from build123d import *

# Parameters (mm, degrees)
EXTRUDE_1_DEPTH     = 12.2
SKETCH_3_W          = 3.6
SKETCH_3_H          = 1.2
CUT_EXTRUDE_1_DEPTH = 2
SKETCH_4_R          = 6.1
SKETCH_4_R_2        = 2.75
EXTRUDE_2_DEPTH     = 4.4
SKETCH_4_3_W        = 6.5
SKETCH_4_3_H        = 9.8
CUT_EXTRUDE_2_DEPTH = 0.2
SKETCH_5_R          = 2.4
SKETCH_5_R_2        = 0.9
EXTRUDE_3_DEPTH     = 3.4
CUT_EXTRUDE_3_REACH = 29.316


with BuildPart() as part:
    # Sketch 1 → Extrude 1 (new body)
    with BuildSketch(Plane.XY):
        Polygon((-11.25, 0), (11.25, 0), (11.25, 15.8), (16.2, 15.8), (16.2, 18.3), (11.25, 18.3), (11.25, 22.3), (-11.25, 22.3), (-11.25, 18.3), (-16.2, 18.3), (-16.2, 15.8), (-11.25, 15.8), align=None)
    extrude(amount=EXTRUDE_1_DEPTH)

    # Sketch 3 → Cut-Extrude 1 (cut)
    with BuildSketch(Plane(origin=(11.25, 0, 0), x_dir=(0, 0, -1), z_dir=(1, 0, 0))):
        with Locations((-6.1, 4.4)):
            Rectangle(SKETCH_3_W, SKETCH_3_H)
    extrude(amount=-CUT_EXTRUDE_1_DEPTH, mode=Mode.SUBTRACT)

    # Sketch 4 → Extrude 2 (add)
    with BuildSketch(Plane(origin=(0, 22.3, 0), x_dir=(1, 0, 0), z_dir=(0, 1, 0))):
        with Locations((5.15, -6.1)):
            Circle(SKETCH_4_R)
        with Locations((-0.6, -6.1)):
            Circle(SKETCH_4_R_2)
    extrude(amount=EXTRUDE_2_DEPTH)

    # Sketch 4_3 → Cut-Extrude 2 (cut)
    with BuildSketch(Plane(origin=(0, 22.3, 0), x_dir=(1, 0, 0), z_dir=(0, 1, 0))):
        with Locations((-6.8, -6.1)):
            Rectangle(SKETCH_4_3_W, SKETCH_4_3_H)
    extrude(amount=-CUT_EXTRUDE_2_DEPTH, mode=Mode.SUBTRACT)

    # Sketch 5 → Extrude 3 (add)
    with BuildSketch(Plane(origin=(0, 26.7, 0), x_dir=(1, 0, 0), z_dir=(0, 1, 0))):
        with Locations(Location((5.15, -6.1, 0), (0, 0, 180))):
            Circle(SKETCH_5_R)
        with Locations(Location((5.15, -6.1, 0), (0, 0, 180))):
            Circle(SKETCH_5_R_2, mode=Mode.SUBTRACT)
    extrude(amount=EXTRUDE_3_DEPTH)

    # Sketch 6 → Cut-Extrude 3 (cut, up to next)
    with BuildSketch(Plane(origin=(0, 18.3, 0), x_dir=(1, 0, 0), z_dir=(0, 1, 0)), mode=Mode.PRIVATE) as cut_extrude_3_sk1:
        with BuildLine():
            Line((-16.2, -6.6), (-15.079795897, -6.6))
            ThreePointArc((-15.079795897, -6.6), (-13, -6.1), (-15.079795897, -5.6))
            Line((-15.079795897, -5.6), (-16.2, -5.6))
            Line((-16.2, -5.6), (-16.2, -6.6))
        make_face()
    cut_extrude_3_tool1 = extrude(cut_extrude_3_sk1.sketch, amount=-CUT_EXTRUDE_3_REACH, mode=Mode.PRIVATE) & part.part
    cut_extrude_3 = cut_extrude_3_tool1.solids().sort_by_distance((-14.439154, 18.3, 6.1))[0]
    add(cut_extrude_3, mode=Mode.SUBTRACT)

    # Mirror 1: Cut-Extrude 3 across plane
    add(cut_extrude_3.mirror(Plane(origin=(0, 0, 0), x_dir=(0, 0, 1), z_dir=(1, 0, 0))), mode=Mode.SUBTRACT)


solid = part.part
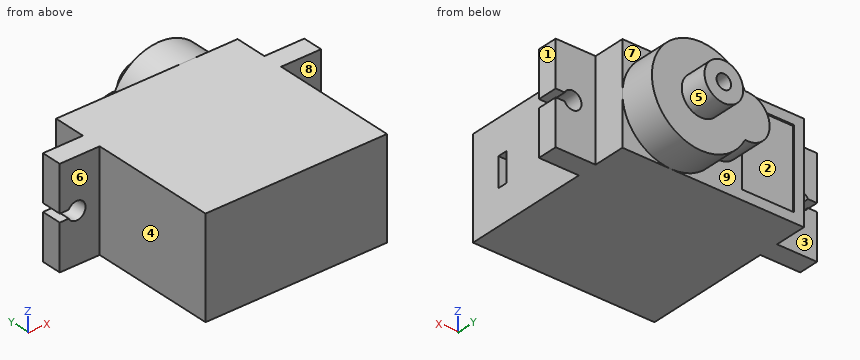
The model under review builds one solid part; all positions refer to its coordinate system, in mm. Face numbers are marked on the shaded views. A direction names the side the tool comes from. Give positions to 0.01 mm unless a question says otherwise; leave off trailing zeros. Loops run counter-clockwise (first coordinate to the right, second up) from the corner with the lowest first, then second, coordinate; pieces in that order, holes last. Notation, with made-up numbers: (-21.75, 17) -> (30.25, 17) arc R25 cw to (30.25, 51) -> close; hole circle Ø8 at (-18, 79.25). An arc over 180 degrees is marked (long way). Put each result on its own line as item: value. Start each with the question number.
1. We need section A-A on x = 14.1. State the section outline as (y, z) points.
2. We need section C-C on y = 14.5. State the section outline as (x, z) points.
3. Wall thickness on probe 1 along Z at (x, y) = (14.1, 16.5); probe 2 along Y at (x, z) = (10, 4.5); probe 3 along Y at (x, z) = (-11, 1.75): over which ranges is each line inside the solid? List them lowest first.
4. For the marked faces 5, 6, 7, 8 and 9, list the 3-axis set-ups (+Z, -Z, +X, -X, +Y, -Y) from which the entire face can be reached by the end or side of a thin tool; tool diameter is ignored.
5. We need section B-B on x = -6. State the section outline as (y, z) points, then the cut area to 3 significant figures.
6. We need section D-D on y = 28. State the section outline as (x, z) points.
7. Clearance check with flat-ended pins moving along their axes: P1, Ø1, axis at x = 10.5, z = 5, coming from the +Y side; P2, Ø2, axis at y = 27, z = 8, coming from the +X side; P3, Ø3, axis at x = -14.1, z = 6.1, coming from the -Y side. State where each tip first meets the part, or that it passes through.
8. Mouldability with a two-part tool opening along X and no side actions: class the marked faces 1, 2, 3 and 4 as released by +X, released by -X, zero draft, split by the parting line, or undercut.
Determined:
1. outline: (15.8, 0) -> (18.3, 0) -> (18.3, 5) -> (15.8, 5) -> close; (15.8, 7.2) -> (18.3, 7.2) -> (18.3, 12.2) -> (15.8, 12.2) -> close
2. outline: (-11.25, 0) -> (11.25, 0) -> (11.25, 12.2) -> (-11.25, 12.2) -> close
3. probe 1: 0 to 5, 7.2 to 12.2
3. probe 2: 0 to 3.8, 5 to 26.7
3. probe 3: 0 to 22.3
4. face 5: +Y
4. face 6: +Z, -Z, -X, -Y
4. face 7: +Z, +X, +Y
4. face 8: +Z, -Z, +X, -Y
4. face 9: -X, +Y
5. outline: (0, 0) -> (22.3, 0) -> (22.3, 1.2) -> (22.1, 1.2) -> (22.1, 11) -> (22.3, 11) -> (22.3, 12.2) -> (0, 12.2) -> close
5. area: 270 mm^2
6. outline: circle Ø4.8 at (5.15, 6.1); hole circle Ø1.8 at (5.15, 6.1)
7. P1: y = 26.7
7. P2: x = 11.18
7. P3: y = 15.8
8. face 1: released by +X
8. face 2: undercut
8. face 3: zero draft
8. face 4: released by -X
